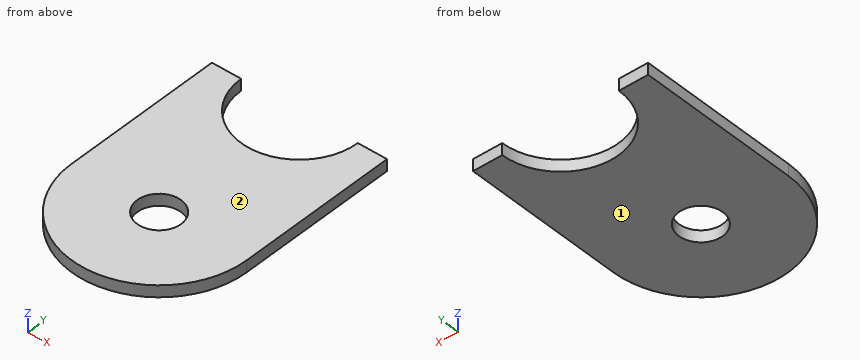
```python
from build123d import *

# Parameters (mm, degrees)
SKETCH1_R           = 4.7625
BOSS_EXTRUDE1_DEPTH = 2.54


with BuildPart() as part:
    # Sketch1 → Boss-Extrude1 (new body)
    with BuildSketch(Plane.XY):
        with BuildLine():
            Line((-19.05, 34.925), (-19.05, -3e-09))
            ThreePointArc((-19.05, -3e-09), (2e-09, -19.05), (19.05, 0))
            Line((19.05, 0), (19.05, 34.925))
            Line((19.05, 34.925), (12.7, 34.925))
            ThreePointArc((12.7, 34.925), (0, 22.225), (-12.7, 34.925))
            Line((-12.7, 34.925), (-19.05, 34.925))
        make_face()
        Circle(SKETCH1_R, mode=Mode.SUBTRACT)
    extrude(amount=BOSS_EXTRUDE1_DEPTH)


solid = part.part
```
Design review of the part built by this model. Coordinates are the model's own, in mm. Face numbers are marked on the shaded views. Round coordinates to 2 decimals unless told otherwise and drop trailing zeros. Write each loop counter-clockwise with the first axis right and the second up, starting at its lowest first coordinate (ties: lowest second). Pieces come first, ordered by that corner, then holes.
Item 1: We need section D-D on x = 9.5. Write out the cut boundary in (y, z), and give its area (3 significant figures).
Item 2: For probe 1 along Y at (x, z) = (1.5, 0.25); probe 2 along X at (y, z) = (3.5, 0.8); probe 3 along X at (y, z) = (-2, 0.3), list the stretches that pass through material, from the lowest coordinate up.
Item 3: Clearance check with flat-ended pins moving along their axes: pin 1 Ø1.5 at (x, z) = (0, 2) entering from -Y; pin 2 Ø1 at (x, z) = (10.5, 1.5) entering from +Y. State where each tip first meets the part, or that it passes through.
Item 4: We need section C-C on y = -2.5. Write out the cut boundary in (x, z).
Item 5: The part is to be moulded in two halves that separate along Z. For the marked faces 1 and 2, say which applies: +Z half, -Z half, draft (parallel to the pull), parting line (faces both ways), or undercut.
Returned:
1. outline: (-16.51, 0) - (26.5, 0) - (26.5, 2.54) - (-16.51, 2.54) - close
1. area: 109 mm2
2. probe 1: y = -18.99 to -4.52, 4.52 to 22.31
2. probe 2: x = -19.05 to -3.23, 3.23 to 19.05
2. probe 3: x = -18.94 to -4.32, 4.32 to 18.94
3. pin 1: stops at y = -19.05
3. pin 2: stops at y = 28.58
4. outline: (-18.89, 0) - (-4.05, 0) - (-4.05, 2.54) - (-18.89, 2.54) - close; (4.05, 0) - (18.89, 0) - (18.89, 2.54) - (4.05, 2.54) - close
5. face 1: -Z half
5. face 2: +Z half
